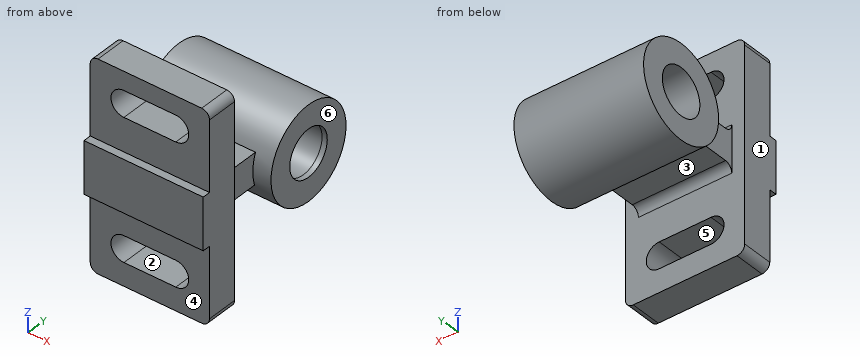
```python
from build123d import *

# Parameters (mm, degrees)
BOSS_EXTRUDE2_DEPTH = 46
FILLET1_R           = 3
CUT_EXTRUDE1_DEPTH  = 46
SKETCH5_R           = 18
SKETCH5_R_2         = 9
BOSS_EXTRUDE3_DEPTH = 50
SKETCH6_R           = 18
SKETCH6_R_2         = 9
BOSS_EXTRUDE4_DEPTH = 2
SKETCH7_R           = 18
SKETCH7_R_2         = 9
CUT_EXTRUDE2_DEPTH  = 2
BOSS_EXTRUDE5_DEPTH = 36
FILLET2_R           = 3


with BuildPart() as part:
    # Sketch3 → Boss-Extrude2 (new body)
    with BuildSketch(Plane(origin=(0, 0, 0), x_dir=(0, 0, -1), z_dir=(1, 0, 0))):
        Polygon((-39.518072289, 0), (-39.518072289, 12), (40.481927711, 12), (40.481927711, 0), (10.481927711, 0), (10.481927711, -3), (-9.518072289, -3), (-9.518072289, 0), align=None)
    extrude(amount=-BOSS_EXTRUDE2_DEPTH)

    # Fillet1
    fillet1_edges = [part.edges().sort_by_distance(p)[0] for p in [
        (-46, 6, -40.481927711),
        (-46, 6, 39.518072289),
        (0, 6, 39.518072289),
        (0, 6, -40.481927711),
    ]]
    fillet(fillet1_edges, radius=FILLET1_R)

    # Sketch4 → Cut-Extrude1 (cut)
    with BuildSketch(Plane(origin=(0, 12, 0), x_dir=(1, 0, 0), z_dir=(0, 1, 0))):
        with BuildLine():
            Line((-33, -22.374092955), (-13, -22.374092955))
            ThreePointArc((-13, -22.374092955), (-8, -27.374092955), (-13, -32.374092955))
            Line((-13, -32.374092955), (-33, -32.374092955))
            ThreePointArc((-33, -32.374092955), (-38, -27.374092955), (-33, -22.374092955))
        make_face()
        with BuildLine():
            Line((-33, 31.625907045), (-13, 31.625907045))
            ThreePointArc((-13, 31.625907045), (-8, 26.625907045), (-13, 21.625907045))
            Line((-13, 21.625907045), (-33, 21.625907045))
            ThreePointArc((-33, 21.625907045), (-38, 26.625907045), (-33, 31.625907045))
        make_face()
    extrude(amount=-CUT_EXTRUDE1_DEPTH, mode=Mode.SUBTRACT)



with BuildPart() as body_2:
    # Sketch5 → Boss-Extrude3 (new body)
    with BuildSketch(Plane(origin=(0, 0, 0), x_dir=(0, 0, -1), z_dir=(1, 0, 0))):
        with Locations((0.481927711, 45)):
            Circle(SKETCH5_R)
        with Locations((0.481927711, 45)):
            Circle(SKETCH5_R_2, mode=Mode.SUBTRACT)
    extrude(amount=-BOSS_EXTRUDE3_DEPTH)

    # Sketch6 → Boss-Extrude4 (add)
    with BuildSketch(Plane(origin=(0, 0, 0), x_dir=(0, 0, -1), z_dir=(1, 0, 0))):
        with Locations((0.481927711, 45)):
            Circle(SKETCH6_R)
        with Locations((0.481927711, 45)):
            Circle(SKETCH6_R_2, mode=Mode.SUBTRACT)
    extrude(amount=BOSS_EXTRUDE4_DEPTH)

    # Sketch7 → Cut-Extrude2 (cut)
    with BuildSketch(Plane.ZY.offset(50)):
        with Locations(Location((-0.481927711, 45, 0), (0, 0, 180))):
            Circle(SKETCH7_R)
        with Locations(Location((-0.481927711, 45, 0), (0, 0, 180))):
            Circle(SKETCH7_R_2, mode=Mode.SUBTRACT)
    extrude(amount=-CUT_EXTRUDE2_DEPTH, mode=Mode.SUBTRACT)


with BuildPart() as part_1:
    add(part.part)

    add(body_2.part)  # Boss-Extrude5 merges body 2
    # Sketch8 → Boss-Extrude5 (add)
    with BuildSketch(Plane(origin=(-5, 0, 0), x_dir=(0, 0, -1), z_dir=(1, 0, 0))):
        with BuildLine():
            Line((-6.148609037, 28.265724323), (-6.148609037, 12))
            Line((-6.148609037, 12), (5.851390963, 12))
            Line((5.851390963, 12), (5.851390963, 27.819520834))
            ThreePointArc((5.851390963, 27.819520834), (-0.186915304, 27.012430708), (-6.148609037, 28.265724323))
        make_face()
    extrude(amount=-BOSS_EXTRUDE5_DEPTH)

    # Fillet2
    fillet2_edges = [part_1.edges().sort_by_distance(p)[0] for p in [
        (-23, 12, -5.851390963),
        (-23, 12, 6.148609037),
    ]]
    fillet(fillet2_edges, radius=FILLET2_R)


solid = part_1.part
```
Read the model definition and answer for the solid it produces. Units are mm, in the model's axes. Face numbers are marked on the shaded views. A direction names the side the tool comes from. Give positions to 0.01 mm unless a question says otherwise; leave off trailing zeros. Order: outer loops, then holes, each group sorted by start corner. A loop starts at its lowest first (then second) coordinate and runs counter-clockwise, first axis right, second up.
(1) Straight lines are drawn through the part: L1, parallel to Z at x = -35, y = 45; L2, parallel to Z at x = -34, y = 5.5; L3, parallel to Y at x = -26.5, z = 18. For each, find the intervals that lie inside material, in ascending order.
(2) For a pull along X with two mould halves and no side action, classify the marked faces 4, 5 and 6 as released by +X, released by -X, zero draft, split by the parting line, or undercut.
(3) Given pin 1 (15 mm diameter, centred on x = -28.5, z = -21, fed in from -Y); pin 2 (12 mm diameter, centred on x = -37.5, z = -2.5, fed in from +Y); pin 3 (3 mm diameter, centred on x = -33.5, y = 51.5, fed in from -Z); pin 4 (11 mm diameter, centred on y = 45, z = -0.48, fed in from -X), each flat-ended and moving along its own axis, determine where each tip first touches the part or whether it passes through.
(4) Find section A-A (y = 45). Give the vertices of the cut face in (x, z).
(5) Find section D-D (y = 31). Give the vertices of the cut face in (x, z).
(6) Find section B-B (x = -25). Give the vertices of the cut face in (y, z), plus the area to 3 significant figures.
(7) For the marked faces 1, 2 and 3, determine the directions among +Z, -Z, +X, -X, +Y, -Y from which every point of the face is accessible in a straight line to the end or side of a thin tool.
(8) Find section C-C (z = 31). Give the vertices of the cut face in (x, y), plus the area to 3 significant figures.
Result sheet:
1. L1: z = -18.48 to -9.48, 8.52 to 17.52
1. L2: z = -40.48 to -31.52, -21.73 to 22.48, 32.27 to 39.52
1. L3: y = 0 to 12
2. face 4: zero draft
2. face 5: undercut
2. face 6: released by +X
3. pin 1: stops at y = 0
3. pin 2: stops at y = 63
3. pin 3: stops at z = -17.77
3. pin 4: passes through
4. outline: (-48, -18.48) - (2, -18.48) - (2, -9.48) - (-48, -9.48) - close; (-48, 8.52) - (2, 8.52) - (2, 17.52) - (-48, 17.52) - close
5. outline: (-48, -11.8) - (2, -11.8) - (2, 10.83) - (-48, 10.83) - close
6. outline: (-3, -10.48) - (0, -10.48) - (0, -21.63) - (12, -21.63) - (12, -8.85) arc R3 cw to (15, -5.85) - (27.82, -5.85) arc R18 ccw (long way) to (28.27, 6.15) - (15, 6.15) arc R3 cw to (12, 9.15) - (12, 22.37) - (0, 22.37) - (0, 9.52) - (-3, 9.52) - close; (0, -40.48) - (12, -40.48) - (12, -31.63) - (0, -31.63) - close; (0, 32.37) - (12, 32.37) - (12, 39.52) - (0, 39.52) - close; hole circle Ø18 at (45, -0.48)
6. area: 1,730 mm2
7. face 1: +Z, -Z, -X, -Y
7. face 2: +Y, -Y
7. face 3: -Z, +X, -X
8. outline: (-46, 0) - (-36.44, 0) - (-36.44, 12) - (-46, 12) - close; (-9.56, 0) - (0, 0) - (0, 12) - (-9.56, 12) - close
8. area: 229 mm2
